Can you work these out from the model? Positions are in its coordinate system, mm. A direction names the side the tool comes from. Round coordinates to 2 decimals unless told otherwise and drop trailing zeros. Loops run counter-clockwise (first coordinate to the right, second up) from the corner with the lowest first, then second, coordinate; pieces in that order, holes last. Notation, with made-up numbers: (34, 67.25) -> (43, 67.25) arc R11 ccw to (43, 78.25) -> close; hole circle Ø5 at (28, 51.25). An arc over 180 degrees is marked (long way). Write each question's results on one line, items separated by ' | '.
from build123d import *

# Parameters (mm, degrees)
F1_DEPTH = 60
F2_DEPTH = 10


with BuildPart() as f1:
    # F0 (on Front) → F1 (new body)
    with BuildSketch(Plane.XZ):
        with BuildLine():
            Line((250, -205), (250, 20))
            Line((250, 20), (250, 245))
            ThreePointArc((250, 245), (242.67767, 262.67767), (225, 270))
            Line((225, 270), (-225, 270))
            ThreePointArc((-225, 270), (-242.67767, 262.67767), (-250, 245))
            Line((-250, 245), (-250, -205))
            ThreePointArc((-250, -205), (-242.67767, -222.67767), (-225, -230))
            Line((-225, -230), (225, -230))
            ThreePointArc((225, -230), (242.67767, -222.67767), (250, -205))
        make_face()
        with BuildLine():
            Line((245.000005, 20), (245.000005, -205))
            ThreePointArc((245.000005, -205), (239.142139, -219.142139), (225, -225.000005))
            Line((225, -225.000005), (-225, -225.000005))
            ThreePointArc((-225, -225.000005), (-239.142139, -219.142139), (-245.000005, -205))
            Line((-245.000005, -205), (-245.000005, 245))
            ThreePointArc((-245.000005, 245), (-239.142139, 259.142139), (-225, 265.000005))
            Line((-225, 265.000005), (225, 265.000005))
            ThreePointArc((225, 265.000005), (239.142139, 259.142139), (245.000005, 245))
            Line((245.000005, 245), (245.000005, 20))
        make_face(mode=Mode.SUBTRACT)
    extrude(amount=F1_DEPTH)

    # F0 (on Front) → F2 (join)
    with BuildSketch(Plane.XZ):
        with BuildLine():
            ThreePointArc((225, -225.000005), (239.142139, -219.142139), (245.000005, -205))
            Line((245.000005, -205), (245.000005, 20))
            Line((245.000005, 20), (245.000005, 245))
            ThreePointArc((245.000005, 245), (239.142139, 259.142139), (225, 265.000005))
            Line((225, 265.000005), (-225, 265.000005))
            ThreePointArc((-225, 265.000005), (-239.142139, 259.142139), (-245.000005, 245))
            Line((-245.000005, 245), (-245.000005, -205))
            ThreePointArc((-245.000005, -205), (-239.142139, -219.142139), (-225, -225.000005))
            Line((-225, -225.000005), (225, -225.000005))
        make_face()
    extrude(amount=F2_DEPTH)


solid = f1.part
1. We'd pull the mould along X, two halves only. Please class faces 1 (the face through (239.297, -34.65, -218.986)), 2 (the face through (-3, -30, -230)), 3 (the face through (-3, -10, 23)), 4 (the face through (-242.871, -29.58, -222.482)): pulls with the +X half, pulls with the -X half, needs draft (parallel to the pull), parting line crosses it, or undercut.
Final values:
face 1: undercut | face 2: needs draft | face 3: undercut | face 4: pulls with the -X half
2. If we section it at B-B (y = -34): List the corners of the cut face in (x, z) for me.
Final values:
outline: (-250, -205) arc R25 ccw to (-225, -230) -> (225, -230) arc R25 ccw to (250, -205) -> (250, 245) arc R25 ccw to (225, 270) -> (-225, 270) arc R25 ccw to (-250, 245) -> close; hole (-245, -205) arc R20 ccw to (-225, -225) -> (225, -225) arc R20 ccw to (245, -205) -> (245, 245) arc R20 ccw to (225, 265) -> (-225, 265) arc R20 ccw to (-245, 245) -> close
3. On a 3-axis mill with a long thin cutter (end or side, diameter ignored), from which of +Z, -Z, +X, -X, +Y, -Y can I reach the whole of each face in a straight line? I mean faces 5 (the face through (-242.482, -29.58, 262.871)), 6 (the face through (-245, -35, 17)). Say none if no direction works.
Final values:
face 5: +Z, -X, +Y, -Y | face 6: -Y
4. Please list where these lines run through material, in increasing order: line 1 (X direction, y = -14.5, z = 152.5); line 2 (Z direction, x = -204.5, y = -17); line 3 (Y direction, x = 218, z = -7). Write a range as from..to.
Final values:
line 1: -250..-245, 245..250 | line 2: -230..-225, 265..270 | line 3: -10..0
5. Will this pin go through, and if not, where does the flat tip stop? pin 1 (5 mm diameter, centred on x = 136.5, z = -141.5, fed in from +Y).
Final values:
pin 1: y = 0
6. If we section it at A-A (z = -172.5): List the corners of the cut face in (x, y) for me, then the cut area to 3 significant figures.
Final values:
outline: (-250, -60) -> (-245, -60) -> (-245, -10) -> (245, -10) -> (245, -60) -> (250, -60) -> (250, 0) -> (-250, 0) -> close | area: 5,500 mm2
7. If we section it at C-C (x = 98): List the corners of the cut face in (y, z) for me, then the cut area to 3 significant figures.
Final values:
outline: (-60, -230) -> (0, -230) -> (0, 270) -> (-60, 270) -> (-60, 265) -> (-10, 265) -> (-10, -225) -> (-60, -225) -> close | area: 5,500 mm2
